Source: CAD feature listing. Evaluate the final solid. Frame: model axes, mm. A direction names the side the tool comes from. Give positions to 0.01 mm unless a question says otherwise; leave off trailing zeros. Loops run counter-clockwise (first coordinate to the right, second up) from the corner with the lowest first, then second, coordinate; pieces in that order, holes last. Notation, with made-up numbers: (66, 68.25) - (93, 68.25) arc R15 ccw to (93, 80.25) - close; hole circle Ø7 at (-21, 52.25). An arc over 180 degrees is marked (long way). Write each question's results on one line, items separated by ' | '. Start each with the question number.
(1) Cut plane C-C on z = 0.65. Return the cut outline in (x, y), then the cut area to 3 significant figures.
(2) Cut plane A-A on x = 0. Return the cut outline in (y, z).
(3) Cut plane D-D on x = -8. Return the cut outline in (y, z), then the cut area to 3 significant figures.
(4) Reachability of faces 5 (the cylindrical face through (-0.59, -4.46, 2.25)), 6 (the flat face through (-2, -2, 1)), 7 (the flat face through (1, -2, 2.5)) from +Z, -Z, +X, -X, +Y, -Y: full face, straight path, thin tool, end or side. Return the list, or none.
(5) Pull-direction query (X, two-part tool) for faces 1 (the cylindrical face through (-2.38, 10.74, 0.99)), 2 (the flat face through (-3, 3, 0)), 3 (the cylindrical face through (0.55, 8.51, 0.99)), 4 (the cylindrical face through (8.75, 0.03, 0.99)); classes: pulls with the +X half, pulls with the -X half, needs draft (parallel to the pull), parting line crosses it, or undercut.
(6) Contact query for flat-ended pins moving along their axis: pin 1 (6.5 mm diameter, centred on x = 0, y = 0, fed in from -Z); pin 2 (1.4 mm diameter, centred on x = 0, y = -8, fed in from -Z); pin 3 (1.5 mm diameter, centred on y = -4.5, z = 1.5, fed in from -X). Output: stop coordinate, or through.
(7) Material intervals for line 1 along Y through (x, z) = (0, 0.65); line 2 along Y through (x, z) = (0, 1.9); line 3 along Z through (x, y) = (5.25, 9.5), sorted ascending. Write a range as [from, to].
Autodesk Inventor part; units mm, degrees
ref_plane "YZ Plane" through (0, 0, 0) normal (1, 0, 0) x (0, 1, 0)
ref_plane "XZ Plane" through (0, 0, 0) normal (0, 1, 0) x (-1, 0, 0)
ref_plane "XY Plane" through (0, 0, 0) normal (0, 0, 1) x (1, 0, 0)
sketch "Sketch1" plane through (0, 0, 0) normal (0, 0, 1) x (1, 0, 0)
  circle A0 centre (0, 0) radius 11
  dimension "d0" = 22
extrude "Extrusion1" add sketch "Sketch1" along normal blind 2
sketch "Sketch2" plane through (0, 0, 2) normal (0, 0, 1) x (1, 0, 0)
  circle A0 centre (0, 0) radius 4.5
  dimension "d3" = 9
extrude "Extrusion2" add sketch "Sketch2" along normal blind 0.5
sketch "Sketch3" plane through (0, 0, 2.5) normal (0, 0, 1) x (1, 0, 0)
  circle A0 centre (0, 0) radius 2
  dimension "d6" = 4
extrude "Extrusion3" cut sketch "Sketch3" against normal blind 555
sketch "Sketch4" plane through (0, 0, 0) normal (0, 0, -1) x (-1, 0, 0)
  circle A0 centre (0, 0) radius 3.5
  dimension "d9" = 7
extrude "Extrusion4" cut sketch "Sketch4" against normal blind 1
sketch "Sketch5" plane through (0, 0, 0) normal (0, 0, -1) x (-1, 0, 0)
  circle A0 centre (0, -8) radius 0.75
  circle A1 centre (8, 0) radius 0.75
  circle A2 centre (0, 8) radius 0.75
  circle A3 centre (-8, 0) radius 0.75
extrude "Extrusion5" cut sketch "Sketch5" against normal blind 44
properties part number "B11" material "ABS Plastic"
Ans:
1) outline: circle Ø22 at (0, 0); hole circle Ø1.5 at (-8, 0); hole circle Ø7 at (0, 0); hole circle Ø1.5 at (0, -8); hole circle Ø1.5 at (0, 8); hole circle Ø1.5 at (8, 0) | area: 335 mm^2
2) outline: (-11, 0) - (-8.75, 0) - (-8.75, 2) - (-11, 2) - close; (-7.25, 0) - (-3.5, 0) - (-3.5, 1) - (-2, 1) - (-2, 2.5) - (-4.5, 2.5) - (-4.5, 2) - (-7.25, 2) - close; (2, 1) - (3.5, 1) - (3.5, 0) - (7.25, 0) - (7.25, 2) - (4.5, 2) - (4.5, 2.5) - (2, 2.5) - close; (8.75, 0) - (11, 0) - (11, 2) - (8.75, 2) - close
3) outline: (-7.55, 0) - (-0.75, 0) - (-0.75, 2) - (-7.55, 2) - close; (0.75, 0) - (7.55, 0) - (7.55, 2) - (0.75, 2) - close | area: 27.2 mm^2
4) face 5: +Z | face 6: -Z | face 7: +Z, +X, -X, +Y, -Y
5) face 1: parting line crosses it | face 2: needs draft | face 3: undercut | face 4: undercut
6) pin 1: z = 1 | pin 2: through | pin 3: x = -10.34
7) line 1: [-11, -8.75], [-7.25, -3.5], [3.5, 7.25], [8.75, 11] | line 2: [-11, -8.75], [-7.25, -2], [2, 7.25], [8.75, 11] | line 3: [0, 2]
